```python
from build123d import *

# Parameters (mm, degrees)
SALIENTE_EXTRUIR1_DEPTH = 195
CROQUIS2_W              = 22.660700849
CROQUIS2_H              = 95
CORTAR_EXTRUIR1_DEPTH   = 0.7
CORTAR_EXTRUIR3_DEPTH   = 100


with BuildPart() as part:
    # Croquis1 → Saliente-Extruir1 (new body)
    with BuildSketch(Plane.XY):
        Polygon((0, 0), (22, 0), (20, 0.7), (0, 0.7), align=None)
    extrude(amount=SALIENTE_EXTRUIR1_DEPTH)

    # Croquis2 → Cortar-Extruir1 (cut)
    with BuildSketch(Plane.XZ):
        with Locations((11.330350425, 47.5)):
            Rectangle(CROQUIS2_W, CROQUIS2_H)
    extrude(amount=-CORTAR_EXTRUIR1_DEPTH, mode=Mode.SUBTRACT)

    # Croquis3 → Cortar-Extruir3 (cut)
    with BuildSketch(Plane(origin=(0, 0, 95), x_dir=(-1, 0, 0), z_dir=(0, 0, -1))):
        Polygon((0, 0), (0, 0.7), (-4.864557071, 0.7), (-6.864557071, 0), align=None)
    extrude(amount=-CORTAR_EXTRUIR3_DEPTH, mode=Mode.SUBTRACT)


solid = part.part
```
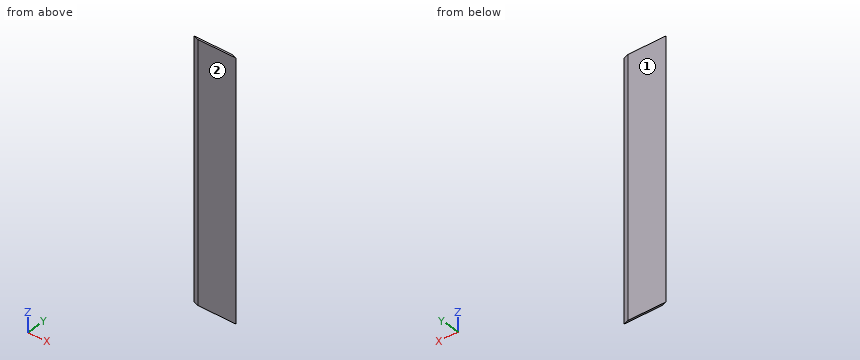
For this review, take the finished solid that the model builds, in its own axes (mm). Face numbers are marked on the shaded views. Round coordinates to 2 decimals unless told otherwise and drop trailing zeros. Write each loop counter-clockwise with the first axis right and the second up, starting at its lowest first coordinate (ties: lowest second). Pieces come first, ordered by that corner, then holes. Notation, with made-up numbers: (50, 69.25) -> (93, 69.25) arc R25 ccw to (93, 103.25) -> close; hole circle Ø9 at (60, -21). An arc over 180 degrees is marked (long way). Use one line per item in the form item = value.
Q1. The part is to be moulded in two halves that separate along Y. For the marked faces 1 and 2, say which applies: released by +Y, released by -Y, zero draft, split by the parting line, or undercut.
Resolved:
face_1 = released by +Y
face_2 = released by -Y
Q2. Clearance check with a flat-ended pin moving along its axis: pin 1 Ø3 at (x, z) = (8, 178) entering from -Y. State where the tip first meets the part, or that it passes through.
Resolved:
pin_1 = 0
Q3. Consider section B-B (y = 0.4). State the section outline as (x, z) points.
Resolved:
outline = (5.72, 95) -> (20.86, 95) -> (20.86, 195) -> (5.72, 195) -> close
Q4. Consider section A-A (z = 156). State the section outline as (x, y) points.
Resolved:
outline = (4.86, 0.7) -> (6.86, 0) -> (22, 0) -> (20, 0.7) -> close
